from build123d import *

# Parameters (mm, degrees)
BOSS_EXTRUDE1_DEPTH      = 4.2418
BOSS_EXTRUDE2_DEPTH      = 8.509
CUT_EXTRUDE1_DEPTH       = 8.509
X_0_397_DIAMETER_HOLE1_D = 3.048
BOSS_EXTRUDE3_DEPTH      = 3.81


with BuildPart() as part:
    # Sketch1 → Boss-Extrude1 (new body)
    with BuildSketch(Plane(origin=(0, 0, 0), x_dir=(0, 0, -1), z_dir=(1, 0, 0))):
        with BuildLine():
            Line((-29.8704, 7.874), (29.8704, 7.874))
            ThreePointArc((29.8704, 7.874), (37.7444, 0), (29.8704, -7.874))
            Line((29.8704, -7.874), (-29.8704, -7.874))
            ThreePointArc((-29.8704, -7.874), (-37.7444, 0), (-29.8704, 7.874))
        make_face()
    extrude(amount=BOSS_EXTRUDE1_DEPTH)

    # Sketch2 → Boss-Extrude2 (add)
    with BuildSketch(Plane(origin=(4.2418, 0, 0), x_dir=(0, 0, -1), z_dir=(1, 0, 0))):
        with BuildLine():
            Line((-21.188107553, 6.604), (21.188107553, 6.604))
            ThreePointArc((21.188107553, 6.604), (23.203225037, 5.61025403), (23.641559152, 3.406599625))
            Line((23.641559152, 3.406599625), (21.463668116, -4.721400375))
            ThreePointArc((21.463668116, -4.721400375), (20.556470547, -6.079117484), (19.010216517, -6.604))
            Line((19.010216517, -6.604), (-19.010216517, -6.604))
            ThreePointArc((-19.010216517, -6.604), (-20.556470547, -6.079117484), (-21.463668116, -4.721400375))
            Line((-21.463668116, -4.721400375), (-23.641559152, 3.406599625))
            ThreePointArc((-23.641559152, 3.406599625), (-23.203225037, 5.61025403), (-21.188107553, 6.604))
        make_face()
    extrude(amount=BOSS_EXTRUDE2_DEPTH)

    # Sketch3 → Cut-Extrude1 (cut)
    with BuildSketch(Plane(origin=(12.7508, 0, 0), x_dir=(0, 0, -1), z_dir=(1, 0, 0))):
        with BuildLine():
            Line((-22.905523672, 3.603819738), (-20.727632636, -4.524180262))
            ThreePointArc((-20.727632636, -4.524180262), (-20.092594338, -5.474582239), (-19.010216517, -5.842))
            Line((-19.010216517, -5.842), (19.010216517, -5.842))
            ThreePointArc((19.010216517, -5.842), (20.092594338, -5.474582239), (20.727632636, -4.524180262))
            Line((20.727632636, -4.524180262), (22.905523672, 3.603819738))
            ThreePointArc((22.905523672, 3.603819738), (22.598689792, 5.146377821), (21.188107553, 5.842))
            Line((21.188107553, 5.842), (-21.188107553, 5.842))
            ThreePointArc((-21.188107553, 5.842), (-22.598689792, 5.146377821), (-22.905523672, 3.603819738))
        make_face()
    extrude(amount=-CUT_EXTRUDE1_DEPTH, mode=Mode.SUBTRACT)

    # X (0.397) Diameter Hole1 (through all)
    with Locations(Plane(origin=(4.2418, 0, 0), x_dir=(0, 0, -1), z_dir=(1, 0, 0))):
        with Locations((-29.8704, 0), (29.8704, 0)):
            Hole(X_0_397_DIAMETER_HOLE1_D / 2)

    # Sketch7 → Boss-Extrude3 (add)
    with BuildSketch(Plane.ZY):
        with BuildLine():
            Line((-22.786295813, 5.334), (22.786295813, 5.334))
            ThreePointArc((22.786295813, 5.334), (28.120295813, 0), (22.786295813, -5.334))
            Line((22.786295813, -5.334), (-22.786295813, -5.334))
            ThreePointArc((-22.786295813, -5.334), (-28.120295813, 0), (-22.786295813, 5.334))
        make_face()
    extrude(amount=BOSS_EXTRUDE3_DEPTH)


solid = part.part
Geometry: final body of the model. Coordinates: model frame, mm. A direction names the side the tool comes from. Give positions to 0.01 mm unless a question says otherwise; leave off trailing zeros. Loops run counter-clockwise (first coordinate to the right, second up) from the corner with the lowest first, then second, coordinate; pieces in that order, holes last. Notation, with made-up numbers: (56, 34) - (95, 34) arc R15 cw to (95, 48) - close; hole circle Ø4 at (75.25, 37.25). An arc over 180 degrees is marked (long way). Answer as CSV lines item,"result". Start each with the question number.
1. Section C-C, the plane y = 0. Return loops of the section in (x, z), plus the area to 3 significant figures.
2. Section D-D, the plane x = -1. Return loops of the section in (y, z), plus the area to 3 significant figures.
3. Reachability of faces 1 (the face through (-2, -5.334, 0)), 2 (the face through (-1.88, -0.12, -28.12)), 3 (the face through (-2, 5.334, 0)), 4 (the face through (8.56, -5.46, 20.11)) from +Z, -Z, +X, -X, +Y, -Y: full face, straight path, thin tool, end or side. Return the list, or none.
4. Pin query (flat end, axial travel): P1, Ø4, axis at y = 0, z = -29.87, coming from the +X side; P2, Ø9.5, axis at x = 10.5, z = -2, coming from the -Y side; P3, Ø7, axis at x = 10, z = -8.5, coming from the +Y side; P4, Ø1.8, axis at y = 0, z = 29.87, coming from the -X side. Return the tip coordinate at first contact, or that it passes through.
5. Section B-B, the plane z = -17. Return loops of the section in (x, y), plus the area to 3 significant figures.
6. Section A-A, the plane x = 8.5. Return loops of the section in (y, z).
7. Ray query, L1, parallel to Y at x = 10, z = 13; L2, parallel to X at y = -3.75, z = 14; L3, parallel to Z at x = 10.75, y = 4.25. Return the intervals inside material, ascending.
Answers:
1,outline,"(-3.81, -28.12) - (0, -28.12) - (0, -28.35) - (4.24, -28.35) - (4.24, -22.73) - (12.75, -22.73) - (12.75, -21.94) - (4.24, -21.94) - (4.24, 21.94) - (12.75, 21.94) - (12.75, 22.73) - (4.24, 22.73) - (4.24, 28.35) - (0, 28.35) - (0, 28.12) - (-3.81, 28.12) - close; (0, -37.74) - (4.24, -37.74) - (4.24, -31.39) - (0, -31.39) - close; (0, 31.39) - (4.24, 31.39) - (4.24, 37.74) - (0, 37.74) - close"
1,area,"522 mm2"
2,outline,"(-5.33, -22.79) arc R5.33 ccw to (5.33, -22.79) - (5.33, 22.79) arc R5.33 ccw to (-5.33, 22.79) - close"
2,area,"576 mm2"
3,face 1,"+Z, -Z, -X, -Y"
3,face 2,"-Z, -X"
3,face 3,"+Z, -Z, -X, +Y"
3,face 4,"+X"
4,P1,"stops at x = 4.24"
4,P2,"stops at y = -6.6"
4,P3,"stops at y = 6.6"
4,P4,"passes through"
5,outline,"(-3.81, -5.33) - (0, -5.33) - (0, -7.87) - (4.24, -7.87) - (4.24, -6.6) - (12.75, -6.6) - (12.75, -5.84) - (4.24, -5.84) - (4.24, 5.84) - (12.75, 5.84) - (12.75, 6.6) - (4.24, 6.6) - (4.24, 7.87) - (0, 7.87) - (0, 5.33) - (-3.81, 5.33) - close"
5,area,"120 mm2"
6,outline,"(-6.6, -19.01) arc R2.54 ccw to (-4.72, -21.46) - (3.41, -23.64) arc R2.54 ccw to (6.6, -21.19) - (6.6, 21.19) arc R2.54 ccw to (3.41, 23.64) - (-4.72, 21.46) arc R2.54 ccw to (-6.6, 19.01) - close; hole (-5.84, -19.01) arc R1.78 ccw to (-4.52, -20.73) - (3.6, -22.91) arc R1.78 ccw to (5.84, -21.19) - (5.84, 21.19) arc R1.78 ccw to (3.6, 22.91) - (-4.52, 20.73) arc R1.78 ccw to (-5.84, 19.01) - close"
7,L1,"y = -6.6 to -5.84, 5.84 to 6.6"
7,L2,"x = -3.81 to 4.24"
7,L3,"z = -23.72 to -22.96, 22.96 to 23.72"
